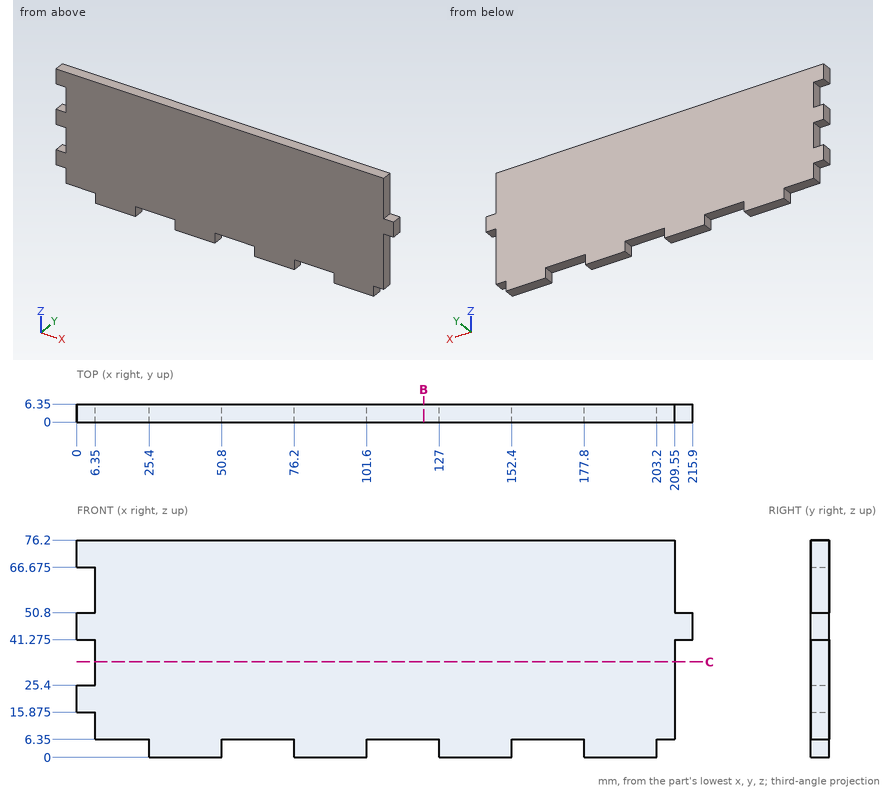
Check sheet for the drawn part. Datum: minimum x, y, z corner. Units: mm. Round coordinates to 2 decimals unless told otherwise and drop trailing zeros. Loops run counter-clockwise (first coordinate to the right, second up) from the corner with the lowest first, then second, coordinate; pieces in that order, holes last. Notation, with made-up numbers: (36.5, -31.5) - (50.5, -31.5) arc R35 cw to (50.5, 1.5) - close; hole circle Ø4 at (51, -11.5). An arc over 180 degrees is marked (long way). Use one line per item in the form item = value.
1. Section check C-C on z = 33.5. Record the cut outline in (x, y).
A:
outline = (6.35, 0) - (209.55, 0) - (209.55, 6.35) - (6.35, 6.35) - close
2. Scan lines: probe 1 along X at (y, z) = (2.5, 26); probe 2 along Z at (x, y) = (56, 5.5); probe 3 along X at (y, z) = (5.5, 71.5). Record each from-to range of solid material in increasing order.
A:
probe_1 = 6.35 to 209.55
probe_2 = 6.35 to 76.2
probe_3 = 0 to 209.55
3. Section check B-B on x = 121.5. Record the cut outline in (y, z).
A:
outline = (0, 6.35) - (6.35, 6.35) - (6.35, 76.2) - (0, 76.2) - close
4. Gauge pin test, flat ends, axial feed: pin 1 Ø1.9 at (y, z) = (2.5, 2) entering from -X; pin 2 Ø3 at (x, y) = (12.5, 3.5) entering from -Z; pin 3 Ø1.9 at (y, z) = (4, 12) entering from -X. Record the tip position at first contact, or that the pin passes through.
A:
pin_1 = 25.4
pin_2 = 6.35
pin_3 = 6.35
